Can you work these out from the model? Positions are in its coordinate system, mm. A direction names the side the tool comes from. Give positions to 0.01 mm unless a question says otherwise; leave off trailing zeros. Write each loop counter-clockwise with the first axis right and the second up, starting at its lowest first coordinate (ties: lowest second). Pieces come first, ordered by that corner, then holes. Notation, with made-up numbers: M -9.75,33.25 L 4.25,33.25 A18 ccw 4.25,40.25 Z; hole C 61.5,13 d5. An arc over 180 degrees is marked long. Write each question's results on one line, items separated by ' | '.
from build123d import *

# Parameters (mm, degrees)
F1_DEPTH = 3


with BuildPart() as f1:
    # F0 (on Top) → F1 (new body)
    with BuildSketch(Plane.XY):
        with BuildLine():
            Line((4.5, 50), (-4.5, 50))
            ThreePointArc((-4.5, 50), (-8.035534, 48.535534), (-9.5, 45))
            Line((-9.5, 45), (-9.5, 5))
            ThreePointArc((-9.5, 5), (-8.035534, 1.464466), (-4.5, 0))
            Line((-4.5, 0), (4.5, 0))
            ThreePointArc((4.5, 0), (8.035534, 1.464466), (9.5, 5))
            Line((9.5, 5), (9.5, 45))
            ThreePointArc((9.5, 45), (8.035534, 48.535534), (4.5, 50))
        make_face()
        with BuildLine():
            ThreePointArc((-6.5, 7.95), (-6.676777, 8.376777), (-6.25, 8.2))
            Line((-6.25, 8.2), (6.25, 8.2))
            ThreePointArc((6.25, 8.2), (6.5, 8.45), (6.75, 8.2))
            ThreePointArc((6.75, 8.2), (6.676777, 8.023223), (6.5, 7.95))
            Line((6.5, 7.95), (6.5, 5.25))
            ThreePointArc((6.5, 5.25), (6.676777, 5.176777), (6.75, 5))
            ThreePointArc((6.75, 5), (6.5, 4.75), (6.25, 5))
            Line((6.25, 5), (-6.25, 5))
            ThreePointArc((-6.25, 5), (-6.676777, 4.823223), (-6.5, 5.25))
            Line((-6.5, 5.25), (-6.5, 7.95))
        make_face(mode=Mode.SUBTRACT)
        with BuildLine():
            ThreePointArc((-6.5, 16.95), (-6.676777, 17.376777), (-6.25, 17.2))
            Line((-6.25, 17.2), (6.25, 17.2))
            ThreePointArc((6.25, 17.2), (6.5, 17.45), (6.75, 17.2))
            ThreePointArc((6.75, 17.2), (6.676777, 17.023223), (6.5, 16.95))
            Line((6.5, 16.95), (6.5, 14.25))
            ThreePointArc((6.5, 14.25), (6.676777, 14.176777), (6.75, 14))
            ThreePointArc((6.75, 14), (6.5, 13.75), (6.25, 14))
            Line((6.25, 14), (-6.25, 14))
            ThreePointArc((-6.25, 14), (-6.676777, 13.823223), (-6.5, 14.25))
            Line((-6.5, 14.25), (-6.5, 16.95))
        make_face(mode=Mode.SUBTRACT)
        with BuildLine():
            ThreePointArc((-6.5, 44.75), (-6.676777, 45.176777), (-6.25, 45))
            Line((-6.25, 45), (6.25, 45))
            ThreePointArc((6.25, 45), (6.5, 45.25), (6.75, 45))
            ThreePointArc((6.75, 45), (6.676777, 44.823223), (6.5, 44.75))
            Line((6.5, 44.75), (6.5, 42.05))
            ThreePointArc((6.5, 42.05), (6.676777, 41.976777), (6.75, 41.8))
            ThreePointArc((6.75, 41.8), (6.5, 41.55), (6.25, 41.8))
            Line((6.25, 41.8), (-6.25, 41.8))
            ThreePointArc((-6.25, 41.8), (-6.676777, 41.623223), (-6.5, 42.05))
            Line((-6.5, 42.05), (-6.5, 44.75))
        make_face(mode=Mode.SUBTRACT)
    extrude(amount=F1_DEPTH)


solid = f1.part
Item 1: I want a section at A-A, the plane x = 1.5. Please give me the cut outline in (y, z), and give its area (3 significant figures).
Geometry says:
outline: M 0,0 L 5,0 L 5,3 L 0,3 Z; M 8.2,0 L 14,0 L 14,3 L 8.2,3 Z; M 17.2,0 L 41.8,0 L 41.8,3 L 17.2,3 Z; M 45,0 L 50,0 L 50,3 L 45,3 Z | area: 121 mm2
Item 2: I want a section at C-C, the plane x = 8. Please give me the cut outline in (y, z), and give its area (3 significant figures).
Geometry says:
outline: M 1.43,0 L 48.57,0 L 48.57,3 L 1.43,3 Z | area: 141 mm2
Item 3: For faces 4 (the face through (-6.5, 43, 1)), 5 (the face through (9.5, 25, 1)), which set-ups out of +Z, -Z, +X, -X, +Y, -Y let a thin tool reach every point of the face, with its end or its side?
Geometry says:
face 4: +Z, -Z | face 5: +Z, -Z, +X, +Y, -Y
Item 4: Thinking about a two-plate mould opening in X: for faces 1 (the face through (0, 25, 0)), 2 (the face through (6.5, 43, 1)), 3 (the face through (-9.5, 25, 1)), which applies, +X half, -X half, draft (parallel to the pull), parting line (faces both ways), or undercut?
Geometry says:
face 1: draft | face 2: undercut | face 3: -X half
Item 5: I'm going to push a flat-ended pin straight in: pin 1 (1 mm diameter, centred on x = -6, z = 1.5, fed in from -Y). Where does the tip first touch, or does it pass through?
Geometry says:
pin 1: stops at y = 0.1
Item 6: I want a section at B-B, the plane z = 2.1. Give the number of separate pieces and of enclosed holes in the cut face, and give its area (3 significant figures).
Geometry says:
separate pieces: 1 | enclosed holes: 3 | area: 802 mm2
Item 7: If I drill on line 1 (Y direction, x = 3, z = 2.2); line 2 (X direction, y = 44.5, z = 0.45); line 3 (Y direction, x = -5.5, z = 2.5), over which ranges is the centre line in solid material (lowest first)? Write a range as from..to.
Geometry says:
line 1: y = 0..5, 8.2..14, 17.2..41.8, 45..50 | line 2: x = -9.5..-6.5, 6.5..9.5 | line 3: y = 0.1..5, 8.2..14, 17.2..41.8, 45..49.9
